from build123d import *

# Parameters (mm, degrees)
SKETCH1_W           = 25
SKETCH1_H           = 20
BOSS_EXTRUDE1_DEPTH = 1.6
SKETCH2_W           = 7.477117313
SKETCH2_H           = 20
BOSS_EXTRUDE2_DEPTH = 15
SKETCH3_W           = 11
SKETCH3_H           = 13.40236223
CUT_EXTRUDE1_DEPTH  = 15
SKETCH4_R           = 1.5
CUT_EXTRUDE2_DEPTH  = 15


with BuildPart() as part:
    # Sketch1 → Boss-Extrude1 (new body)
    with BuildSketch(Plane(origin=(0, 0, 0), x_dir=(1, 0, 0), z_dir=(0, 1, 0))):
        Rectangle(SKETCH1_W, SKETCH1_H)
    extrude(amount=BOSS_EXTRUDE1_DEPTH)

    # Sketch2 → Boss-Extrude2 (add)
    with BuildSketch(Plane(origin=(0, 1.6, 0), x_dir=(1, 0, 0), z_dir=(0, 1, 0))):
        with Locations((8.761441343, 0)):
            Rectangle(SKETCH2_W, SKETCH2_H)
    extrude(amount=BOSS_EXTRUDE2_DEPTH)

    # Sketch3 → Cut-Extrude1 (cut)
    with BuildSketch(Plane(origin=(12.5, 0, 0), x_dir=(0, 0, -1), z_dir=(1, 0, 0))):
        with Locations((0, 9.898818885)):
            Rectangle(SKETCH3_W, SKETCH3_H)
    extrude(amount=-CUT_EXTRUDE1_DEPTH, mode=Mode.SUBTRACT)

    # Sketch4 → Cut-Extrude2 (cut)
    with BuildSketch(Plane(origin=(0, 1.6, 0), x_dir=(1, 0, 0), z_dir=(0, 1, 0))):
        with Locations((-10.1, 7.6)):
            Circle(SKETCH4_R)
        with Locations((-10.1, -7.6)):
            Circle(SKETCH4_R)
    extrude(amount=-CUT_EXTRUDE2_DEPTH, mode=Mode.SUBTRACT)


solid = part.part
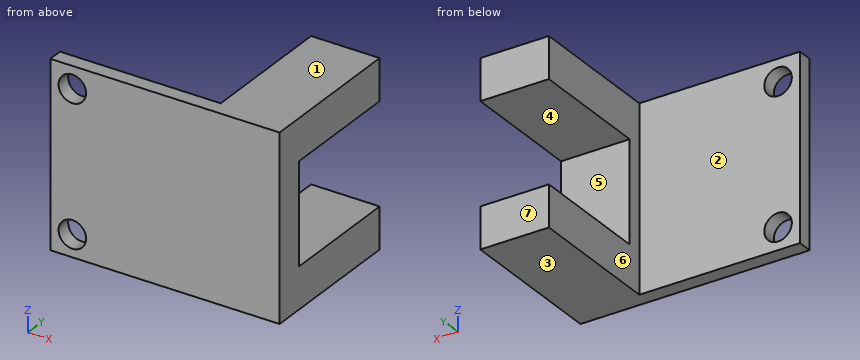
Work out the finished part from the listing and answer in its coordinate system (mm). Face numbers are marked on the shaded views. A direction names the side the tool comes from. Round coordinates to 2 decimals unless told otherwise and drop trailing zeros. Write each loop counter-clockwise with the first axis right and the second up, starting at its lowest first coordinate (ties: lowest second). Pieces come first, ordered by that corner, then holes.
1) The mould has two halves that part along Z. Classify the marked faces 1, 2, 3 and 4: pulls with the +Z half, pulls with the -Z half, needs draft (parallel to the pull), parting line crosses it, or undercut.
2) Given pin 1 Ø6 at (x, z) = (10.5, -1.5) entering from +Y; pin 2 Ø4 at (x, z) = (-10.1, -7.6) entering from -Y; pin 3 Ø10 at (x, z) = (-1.5, -7.5) entering from +Y; pin 4 Ø7.5 at (y, z) = (8.5, 4.5) entering from -X, each flat-ended and moving along its own axis, determine where each tip first touches the part or whether it passes through.
3) A cutting plane is placed at A-A (y = 9). Give the vertices of the cut face in (x, z), plus the area to 3 significant figures.
4) Straight lines are drawn through the part: line 1 (Z direction, x = -10.1, y = 1.25); line 2 (X direction, y = 0.4, z = 7.6); line 3 (Z direction, x = 5.75, y = 5). For each, find the intervals that lie inside material, in ascending order.
5) A cutting plane is placed at B-B (x = -10.1). Give the vertices of the cut face in (y, z).
6) A cutting plane is placed at C-C (z = -7.6). Give the vertices of the cut face in (x, y).
7) A tool of negligible diameter and unlimited length cuts with its end or side. For the marked faces 5, 6 and 7, from which of +Z, -Z, +X, -X, +Y, -Y can it reach the whole face along a straight path? Write none if from no direction.
8) A cutting plane is placed at D-D (x = 9.5). Give the vertices of the cut face in (y, z).
Completed:
1. face 1: pulls with the +Z half
1. face 2: needs draft
1. face 3: pulls with the -Z half
1. face 4: undercut
2. pin 1: stops at y = 3.2
2. pin 2: stops at y = 0
2. pin 3: stops at y = 1.6
2. pin 4: stops at x = 5.02
3. outline: (5.02, -10) - (12.5, -10) - (12.5, -5.5) - (5.02, -5.5) - close; (5.02, 5.5) - (12.5, 5.5) - (12.5, 10) - (5.02, 10) - close
3. area: 67.3 mm2
4. line 1: z = -10 to -9.1, -6.1 to 6.1, 9.1 to 10
4. line 2: x = -12.5 to -11.6, -8.6 to 12.5
4. line 3: z = -10 to -5.5, 5.5 to 10
5. outline: (0, -10) - (1.6, -10) - (1.6, -9.1) - (0, -9.1) - close; (0, -6.1) - (1.6, -6.1) - (1.6, 6.1) - (0, 6.1) - close; (0, 9.1) - (1.6, 9.1) - (1.6, 10) - (0, 10) - close
6. outline: (-12.5, 0) - (-11.6, 0) - (-11.6, 1.6) - (-12.5, 1.6) - close; (-8.6, 0) - (12.5, 0) - (12.5, 16.6) - (5.02, 16.6) - (5.02, 1.6) - (-8.6, 1.6) - close
7. face 5: +X, -X, +Y
7. face 6: +Z, -Z, -X, +Y
7. face 7: +Z, -Z, +X, -X, +Y
8. outline: (0, -10) - (16.6, -10) - (16.6, -5.5) - (3.2, -5.5) - (3.2, 5.5) - (16.6, 5.5) - (16.6, 10) - (0, 10) - close
